Geometry: final body of the model. Coordinates: model frame, mm. Give positions to 0.01 mm unless a question says otherwise; leave off trailing zeros. Write each loop counter-clockwise with the first axis right and the second up, starting at its lowest first coordinate (ties: lowest second). Pieces come first, ordered by that corner, then holes. Notation, with made-up numbers: (26.5, -36.5) - (63.5, -36.5) arc R20 ccw to (63.5, -28.5) - close; hole circle Ø11 at (-30, 66). An arc over 180 degrees is marked (long way). Use CSV: the item, a comma, the result in double quotes. Start each with the question number.
(1) Section A-A on x = 345. Output: boundary loops of the cut face in (y, z), and give its area (4 significant figures).
(2) Line query: probe 1 along Y at (x, z) = (303, 1.95); probe 2 along X at (y, z) = (219.5, 2.3); probe 3 along Y at (x, z) = (264.5, 0.25). Output: solid intervals per line, ascending. Write a range as [from, to].
(3) Section C-C on x = 265.5. Output: boundary loops of the cut face in (y, z), and give its area (3 significant figures).
(4) Section B-B on y = 212.75. Output: boundary loops of the cut face in (x, z).
(5) Section D-D on z = 1.7. Count the separate pieces of the cut face and the enclosed holes in it, and give its area (3 significant figures).
(6) Draft query along Y for faces 1 (the flat face through (333, 219.742, 1)), 2 (the flat face through (314.929, 216, 1)), 3 (the cylindrical face through (354.324, 216.256, 1.479)). Return one class per face: released by +Y, released by -Y, zero draft, split by the parting line, or undercut.
from build123d import *

# Parameters (mm, degrees)
MODEL_R                 = 1.5
SALIENTE_EXTRUIR1_DEPTH = 3


with BuildPart() as part:
    # Model → Saliente-Extruir1 (new body)
    with BuildSketch(Plane.XY):
        with BuildLine():
            Line((256.429131311, 228.742243614), (355.429131311, 228.742243614))
            ThreePointArc((355.429131311, 228.742243614), (358.611111826, 227.424224129), (359.929131311, 224.242243614))
            Line((359.929131311, 224.242243614), (359.929131311, 215.242243614))
            ThreePointArc((359.929131311, 215.242243614), (355.429131311, 210.742243614), (350.929131311, 215.242243614))
            Line((350.929131311, 215.242243614), (350.929131311, 217.492243614))
            Line((350.929131311, 217.492243614), (348.679131311, 219.742243614))
            Line((348.679131311, 219.742243614), (317.179131311, 219.742243614))
            Line((317.179131311, 219.742243614), (314.929131311, 217.492243614))
            Line((314.929131311, 217.492243614), (314.929131311, 215.242243614))
            ThreePointArc((314.929131311, 215.242243614), (313.611111826, 212.060263099), (310.429131311, 210.742243614))
            Line((310.429131311, 210.742243614), (256.429131311, 210.742243614))
            ThreePointArc((256.429131311, 210.742243614), (253.247150795, 212.060263099), (251.929131311, 215.242243614))
            Line((251.929131311, 215.242243614), (251.929131311, 224.242243614))
            ThreePointArc((251.929131311, 224.242243614), (253.247150795, 227.424224129), (256.429131311, 228.742243614))
        make_face()
        with Locations((310.429131311, 215.242243614)):
            Circle(MODEL_R, mode=Mode.SUBTRACT)
        with Locations((292.429131311, 215.242243614)):
            Circle(MODEL_R, mode=Mode.SUBTRACT)
        with Locations((301.429131311, 215.242243614)):
            Circle(MODEL_R, mode=Mode.SUBTRACT)
        with Locations((274.429131311, 215.242243614)):
            Circle(MODEL_R, mode=Mode.SUBTRACT)
        with Locations((283.429131311, 215.242243614)):
            Circle(MODEL_R, mode=Mode.SUBTRACT)
        with Locations((265.429131311, 215.242243614)):
            Circle(MODEL_R, mode=Mode.SUBTRACT)
        with Locations((256.429131311, 215.242243614)):
            Circle(MODEL_R, mode=Mode.SUBTRACT)
        with Locations((355.429131311, 215.242243614)):
            Circle(MODEL_R, mode=Mode.SUBTRACT)
        with BuildLine():
            Line((267.929131311, 222.617243614), (262.929131311, 222.617243614))
            ThreePointArc((262.929131311, 222.617243614), (262.398801225, 222.836913528), (262.179131311, 223.367243614))
            Line((262.179131311, 223.367243614), (262.179131311, 225.117243614))
            ThreePointArc((262.179131311, 225.117243614), (262.398801225, 225.6475737), (262.929131311, 225.867243614))
            Line((262.929131311, 225.867243614), (267.929131311, 225.867243614))
            ThreePointArc((267.929131311, 225.867243614), (268.459461397, 225.6475737), (268.679131311, 225.117243614))
            Line((268.679131311, 225.117243614), (268.679131311, 223.367243614))
            ThreePointArc((268.679131311, 223.367243614), (268.459461397, 222.836913528), (267.929131311, 222.617243614))
        make_face(mode=Mode.SUBTRACT)
        with BuildLine():
            Line((285.929131311, 222.617243614), (280.929131311, 222.617243614))
            ThreePointArc((280.929131311, 222.617243614), (280.398801225, 222.836913528), (280.179131311, 223.367243614))
            Line((280.179131311, 223.367243614), (280.179131311, 225.117243614))
            ThreePointArc((280.179131311, 225.117243614), (280.398801225, 225.6475737), (280.929131311, 225.867243614))
            Line((280.929131311, 225.867243614), (285.929131311, 225.867243614))
            ThreePointArc((285.929131311, 225.867243614), (286.459461397, 225.6475737), (286.679131311, 225.117243614))
            Line((286.679131311, 225.117243614), (286.679131311, 223.367243614))
            ThreePointArc((286.679131311, 223.367243614), (286.459461397, 222.836913528), (285.929131311, 222.617243614))
        make_face(mode=Mode.SUBTRACT)
        with BuildLine():
            Line((258.929131311, 222.617243614), (253.929131311, 222.617243614))
            ThreePointArc((253.929131311, 222.617243614), (253.398801225, 222.836913528), (253.179131311, 223.367243614))
            Line((253.179131311, 223.367243614), (253.179131311, 225.117243614))
            ThreePointArc((253.179131311, 225.117243614), (253.398801225, 225.6475737), (253.929131311, 225.867243614))
            Line((253.929131311, 225.867243614), (258.929131311, 225.867243614))
            ThreePointArc((258.929131311, 225.867243614), (259.459461397, 225.6475737), (259.679131311, 225.117243614))
            Line((259.679131311, 225.117243614), (259.679131311, 223.367243614))
            ThreePointArc((259.679131311, 223.367243614), (259.459461397, 222.836913528), (258.929131311, 222.617243614))
        make_face(mode=Mode.SUBTRACT)
        with BuildLine():
            Line((276.929131311, 222.617243614), (271.929131311, 222.617243614))
            ThreePointArc((271.929131311, 222.617243614), (271.398801225, 222.836913528), (271.179131311, 223.367243614))
            Line((271.179131311, 223.367243614), (271.179131311, 225.117243614))
            ThreePointArc((271.179131311, 225.117243614), (271.398801225, 225.6475737), (271.929131311, 225.867243614))
            Line((271.929131311, 225.867243614), (276.929131311, 225.867243614))
            ThreePointArc((276.929131311, 225.867243614), (277.459461397, 225.6475737), (277.679131311, 225.117243614))
            Line((277.679131311, 225.117243614), (277.679131311, 223.367243614))
            ThreePointArc((277.679131311, 223.367243614), (277.459461397, 222.836913528), (276.929131311, 222.617243614))
        make_face(mode=Mode.SUBTRACT)
        with BuildLine():
            Line((294.929131311, 222.617243614), (289.929131311, 222.617243614))
            ThreePointArc((289.929131311, 222.617243614), (289.398801225, 222.836913528), (289.179131311, 223.367243614))
            Line((289.179131311, 223.367243614), (289.179131311, 225.117243614))
            ThreePointArc((289.179131311, 225.117243614), (289.398801225, 225.6475737), (289.929131311, 225.867243614))
            Line((289.929131311, 225.867243614), (294.929131311, 225.867243614))
            ThreePointArc((294.929131311, 225.867243614), (295.459461397, 225.6475737), (295.679131311, 225.117243614))
            Line((295.679131311, 225.117243614), (295.679131311, 223.367243614))
            ThreePointArc((295.679131311, 223.367243614), (295.459461397, 222.836913528), (294.929131311, 222.617243614))
        make_face(mode=Mode.SUBTRACT)
        with BuildLine():
            Line((303.929131311, 222.617243614), (298.929131311, 222.617243614))
            ThreePointArc((298.929131311, 222.617243614), (298.398801225, 222.836913528), (298.179131311, 223.367243614))
            Line((298.179131311, 223.367243614), (298.179131311, 225.117243614))
            ThreePointArc((298.179131311, 225.117243614), (298.398801225, 225.6475737), (298.929131311, 225.867243614))
            Line((298.929131311, 225.867243614), (303.929131311, 225.867243614))
            ThreePointArc((303.929131311, 225.867243614), (304.459461397, 225.6475737), (304.679131311, 225.117243614))
            Line((304.679131311, 225.117243614), (304.679131311, 223.367243614))
            ThreePointArc((304.679131311, 223.367243614), (304.459461397, 222.836913528), (303.929131311, 222.617243614))
        make_face(mode=Mode.SUBTRACT)
        with BuildLine():
            Line((321.929131311, 222.617243614), (316.929131311, 222.617243614))
            ThreePointArc((316.929131311, 222.617243614), (316.398801225, 222.836913528), (316.179131311, 223.367243614))
            Line((316.179131311, 223.367243614), (316.179131311, 225.117243614))
            ThreePointArc((316.179131311, 225.117243614), (316.398801225, 225.6475737), (316.929131311, 225.867243614))
            Line((316.929131311, 225.867243614), (321.929131311, 225.867243614))
            ThreePointArc((321.929131311, 225.867243614), (322.459461397, 225.6475737), (322.679131311, 225.117243614))
            Line((322.679131311, 225.117243614), (322.679131311, 223.367243614))
            ThreePointArc((322.679131311, 223.367243614), (322.459461397, 222.836913528), (321.929131311, 222.617243614))
        make_face(mode=Mode.SUBTRACT)
        with BuildLine():
            Line((312.929131311, 222.617243614), (307.929131311, 222.617243614))
            ThreePointArc((307.929131311, 222.617243614), (307.398801225, 222.836913528), (307.179131311, 223.367243614))
            Line((307.179131311, 223.367243614), (307.179131311, 225.117243614))
            ThreePointArc((307.179131311, 225.117243614), (307.398801225, 225.6475737), (307.929131311, 225.867243614))
            Line((307.929131311, 225.867243614), (312.929131311, 225.867243614))
            ThreePointArc((312.929131311, 225.867243614), (313.459461397, 225.6475737), (313.679131311, 225.117243614))
            Line((313.679131311, 225.117243614), (313.679131311, 223.367243614))
            ThreePointArc((313.679131311, 223.367243614), (313.459461397, 222.836913528), (312.929131311, 222.617243614))
        make_face(mode=Mode.SUBTRACT)
        with BuildLine():
            Line((357.929131311, 222.617243614), (352.929131311, 222.617243614))
            ThreePointArc((352.929131311, 222.617243614), (352.398801225, 222.836913528), (352.179131311, 223.367243614))
            Line((352.179131311, 223.367243614), (352.179131311, 225.117243614))
            ThreePointArc((352.179131311, 225.117243614), (352.398801225, 225.6475737), (352.929131311, 225.867243614))
            Line((352.929131311, 225.867243614), (357.929131311, 225.867243614))
            ThreePointArc((357.929131311, 225.867243614), (358.459461397, 225.6475737), (358.679131311, 225.117243614))
            Line((358.679131311, 225.117243614), (358.679131311, 223.367243614))
            ThreePointArc((358.679131311, 223.367243614), (358.459461397, 222.836913528), (357.929131311, 222.617243614))
        make_face(mode=Mode.SUBTRACT)
        with BuildLine():
            Line((348.929131311, 222.617243614), (343.929131311, 222.617243614))
            ThreePointArc((343.929131311, 222.617243614), (343.398801225, 222.836913528), (343.179131311, 223.367243614))
            Line((343.179131311, 223.367243614), (343.179131311, 225.117243614))
            ThreePointArc((343.179131311, 225.117243614), (343.398801225, 225.6475737), (343.929131311, 225.867243614))
            Line((343.929131311, 225.867243614), (348.929131311, 225.867243614))
            ThreePointArc((348.929131311, 225.867243614), (349.459461397, 225.6475737), (349.679131311, 225.117243614))
            Line((349.679131311, 225.117243614), (349.679131311, 223.367243614))
            ThreePointArc((349.679131311, 223.367243614), (349.459461397, 222.836913528), (348.929131311, 222.617243614))
        make_face(mode=Mode.SUBTRACT)
        with BuildLine():
            Line((339.929131311, 222.617243614), (334.929131311, 222.617243614))
            ThreePointArc((334.929131311, 222.617243614), (334.398801225, 222.836913528), (334.179131311, 223.367243614))
            Line((334.179131311, 223.367243614), (334.179131311, 225.117243614))
            ThreePointArc((334.179131311, 225.117243614), (334.398801225, 225.6475737), (334.929131311, 225.867243614))
            Line((334.929131311, 225.867243614), (339.929131311, 225.867243614))
            ThreePointArc((339.929131311, 225.867243614), (340.459461397, 225.6475737), (340.679131311, 225.117243614))
            Line((340.679131311, 225.117243614), (340.679131311, 223.367243614))
            ThreePointArc((340.679131311, 223.367243614), (340.459461397, 222.836913528), (339.929131311, 222.617243614))
        make_face(mode=Mode.SUBTRACT)
        with BuildLine():
            Line((330.929131311, 222.617243614), (325.929131311, 222.617243614))
            ThreePointArc((325.929131311, 222.617243614), (325.398801225, 222.836913528), (325.179131311, 223.367243614))
            Line((325.179131311, 223.367243614), (325.179131311, 225.117243614))
            ThreePointArc((325.179131311, 225.117243614), (325.398801225, 225.6475737), (325.929131311, 225.867243614))
            Line((325.929131311, 225.867243614), (330.929131311, 225.867243614))
            ThreePointArc((330.929131311, 225.867243614), (331.459461397, 225.6475737), (331.679131311, 225.117243614))
            Line((331.679131311, 225.117243614), (331.679131311, 223.367243614))
            ThreePointArc((331.679131311, 223.367243614), (331.459461397, 222.836913528), (330.929131311, 222.617243614))
        make_face(mode=Mode.SUBTRACT)
    extrude(amount=SALIENTE_EXTRUIR1_DEPTH)


solid = part.part
Check values:
1,outline,"(219.74, 0) - (222.62, 0) - (222.62, 3) - (219.74, 3) - close; (225.87, 0) - (228.74, 0) - (228.74, 3) - (225.87, 3) - close"
1,area,"17.25 mm²"
2,probe 1,"y = [210.74, 222.62], [225.87, 228.74]"
2,probe 2,"x = [251.93, 316.94], [348.92, 359.93]"
2,probe 3,"y = [210.74, 214.06], [216.42, 222.62], [225.87, 228.74]"
3,outline,"(210.74, 0) - (213.74, 0) - (213.74, 3) - (210.74, 3) - close; (216.74, 0) - (222.62, 0) - (222.62, 3) - (216.74, 3) - close; (225.87, 0) - (228.74, 0) - (228.74, 3) - (225.87, 3) - close"
3,area,"35.3 mm²"
4,outline,"(252.68, 0) - (314.18, 0) - (314.18, 3) - (252.68, 3) - close; (351.68, 0) - (359.18, 0) - (359.18, 3) - (351.68, 3) - close"
5,separate pieces,"1"
5,enclosed holes,"20"
5,area,"1,290 mm²"
6,face 1,"released by -Y"
6,face 2,"zero draft"
6,face 3,"undercut"
